Design review of the part built by this model. Coordinates are the model's own, in mm. Coordinates: 2 decimals unless noted, no trailing zeros. Loops run counter-clockwise (first coordinate to the right, second up) from the corner with the lowest first, then second, coordinate; pieces in that order, holes last. Notation, with made-up numbers: (7, 83) - (62, 83) arc R26 ccw to (62, 104) - close; hole circle Ø11 at (-9.5, 65.5). An arc over 180 degrees is marked (long way). Answer in a Markdown table with one row per item. Add a question column.
(1) To check wall thickness, follow L1, parallel to X at y = 0.9, z = 0; L2, parallel to X at y = 2.55, z = 8; L3, parallel to X at y = 0.85, z = 27.5. State the ranges of each line that lie inside material, in increasing order. Write a range as [from, to].
(2) We need section B-B, the plane z = 0. Write out the cut boundary in (x, y) (3 decimals).
(3) Clearance check with flat-ended pins moving along their axes: pin 1 (6 mm diameter, centred on x = 0, z = 0, fed in from +Y) (3 decimals); pin 2 (1.5 mm diameter, centred on y = 2.5, z = 23.5, fed in from -X). State where each tip first meets the part, or that it passes through.
(4) We need section C-C, the plane x = -75. Write out the cut boundary in (y, z) (3 decimals), plus the area to 3 significant figures.
(5) We need section A-A, the plane y = 2.4. Write out the cut boundary in (x, z).
(6) We need section D-D, the plane z = 12.5. Write out the cut boundary in (x, y) (3 decimals), plus the area to 3 significant figures.
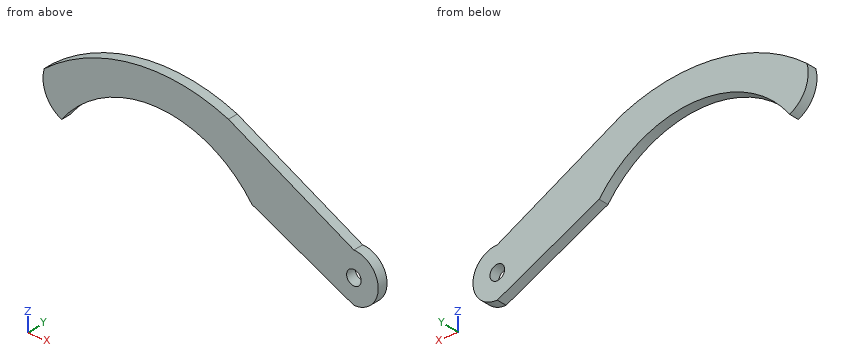
from build123d import *

# Parameters (mm, degrees)
SKETCH1_R           = 2.286
BOSS_EXTRUDE1_DEPTH = 3.175


with BuildPart() as part:
    # Sketch1 → Boss-Extrude1 (new body)
    with BuildSketch(Plane(origin=(0, 0, 0), x_dir=(1, 0, 0), z_dir=(0, 1, 0))):
        with BuildLine():
            Line((-31.898482314, -7.62), (0, 7.62))
            ThreePointArc((0, 7.62), (7.62, 0), (0, -7.62))
            Line((0, -7.62), (-39.266643524, -28.218839839))
            ThreePointArc((-39.266643524, -28.218839839), (-69.304091982, -31.809710463), (-96.940525037, -19.506449524))
            ThreePointArc((-96.940525037, -19.506449524), (-96.41727765, -12.558332827), (-91.501691991, -7.62))
            ThreePointArc((-91.501691991, -7.62), (-61.700087152, -22.761590746), (-31.898482314, -7.62))
        make_face()
        with Locations(Location((0, 0, 0), (0, 0, 270))):
            Circle(SKETCH1_R, mode=Mode.SUBTRACT)
    extrude(amount=BOSS_EXTRUDE1_DEPTH)


solid = part.part
Responses:
| question | item | result |
|---|---|---|
| 1 | L1 | x = [-15.95, -2.29], [2.29, 7.62] |
| 1 | L2 | x = [-92.24, -91.22], [-32.18, -0.72] |
| 1 | L3 | x = [-84.02, -37.9] |
| 2 | outline | (-15.949, 0) - (-2.286, 0) - (-2.286, 3.175) - (-15.949, 3.175) - close; (2.286, 0) - (7.62, 0) - (7.62, 3.175) - (2.286, 3.175) - close |
| 3 | pin 1 | stops at y = 3.175 |
| 3 | pin 2 | stops at x = -92.58 |
| 4 | outline | (0, 20.281) - (3.175, 20.281) - (3.175, 30.649) - (0, 30.649) - close |
| 4 | area | 32.9 mm2 |
| 5 | outline | (-96.94, 19.51) arc R10.05 ccw to (-91.5, 7.62) arc R36.9 cw to (-31.9, 7.62) - (0, -7.62) arc R7.62 ccw to (0, 7.62) - (-39.27, 28.22) arc R56.93 ccw to start; hole circle Ø4.57 at (0, 0) |
| 6 | outline | (-96.39, 0) - (-87.234, 0) - (-87.234, 3.175) - (-96.39, 3.175) - close; (-36.166, 0) - (-9.303, 0) - (-9.303, 3.175) - (-36.166, 3.175) - close |
| 6 | area | 114 mm2 |
